```python
from build123d import *

# Parameters (mm, degrees)
SKETCH3_W                       = 0.5
SKETCH3_H                       = 1.75
SKETCH3_W_2                     = 1.75
SKETCH3_H_2                     = 0.5
BOSS_EXTRUDE1_DEPTH             = 13
BOSS_EXTRUDE1_DIRECTION_2_REACH = 27.695
SKETCH4_R                       = 0.75
CUT_EXTRUDE2_DEPTH              = 4
BOSS_EXTRUDE2_DEPTH             = 1


with BuildPart() as part:
    # Sketch1 → Revolve1 (revolve)
    with BuildSketch(Plane(origin=(0, 0, 0), x_dir=(0, 0, -1), z_dir=(1, 0, 0))):
        with BuildLine():
            ThreePointArc((-3.5, 4), (-2.474873734, 1.525126266), (0, 0.5))
            Line((0, 0.5), (0, 0))
            Line((0, 0), (0, -8.5))
            Line((0, -8.5), (0, -14.5))
            ThreePointArc((0, -14.5), (-2.956795679, -12.007305936), (-1, -8.671572875))
            Line((-1, -8.671572875), (-1, 0.127016654))
            ThreePointArc((-1, 0.127016654), (-2.197145125, 0.657463044), (-3.158848322, 1.546089391))
            Line((-3.158848322, 1.546089391), (-15, 3))
            Line((-15, 3), (-15, 4))
            Line((-15, 4), (-4, 4))
            Line((-4, 4), (-3.5, 4))
        make_face()
    revolve(axis=Axis((0, 10.634252877, 0), (0, 1, 0)))

    # Sketch3 → Boss-Extrude1 (add)
    with BuildSketch(Plane(origin=(0, 0, 0), x_dir=(1, 0, 0), z_dir=(0, 1, 0))):
        with Locations((0, 1.125)):
            Rectangle(SKETCH3_W, SKETCH3_H)
        with Locations((-1.125, 0)):
            Rectangle(SKETCH3_W_2, SKETCH3_H_2)
        with Locations((1.125, 0)):
            Rectangle(SKETCH3_W_2, SKETCH3_H_2)
        with Locations((0, -1.125)):
            Rectangle(SKETCH3_W, SKETCH3_H)
    extrude(amount=-BOSS_EXTRUDE1_DEPTH)

    # Sketch3 → Boss-Extrude1 direction 2 (add, up to next)
    with BuildSketch(Plane(origin=(0, 0, 0), x_dir=(1, 0, 0), z_dir=(0, 1, 0)), mode=Mode.PRIVATE) as boss_extrude1_direction_2_sk1:
        with Locations((0, 1.125)):
            Rectangle(SKETCH3_W, SKETCH3_H)
    boss_extrude1_direction_2_tool1 = extrude(boss_extrude1_direction_2_sk1.sketch, amount=BOSS_EXTRUDE1_DIRECTION_2_REACH, mode=Mode.PRIVATE) - part.part
    # Sketch3 → Boss-Extrude1 direction 2 (add, up to next)
    with BuildSketch(Plane(origin=(0, 0, 0), x_dir=(1, 0, 0), z_dir=(0, 1, 0)), mode=Mode.PRIVATE) as boss_extrude1_direction_2_sk2:
        with Locations((-1.125, 0)):
            Rectangle(SKETCH3_W_2, SKETCH3_H_2)
    boss_extrude1_direction_2_tool2 = extrude(boss_extrude1_direction_2_sk2.sketch, amount=BOSS_EXTRUDE1_DIRECTION_2_REACH, mode=Mode.PRIVATE) - part.part
    # Sketch3 → Boss-Extrude1 direction 2 (add, up to next)
    with BuildSketch(Plane(origin=(0, 0, 0), x_dir=(1, 0, 0), z_dir=(0, 1, 0)), mode=Mode.PRIVATE) as boss_extrude1_direction_2_sk3:
        with Locations((1.125, 0)):
            Rectangle(SKETCH3_W_2, SKETCH3_H_2)
    boss_extrude1_direction_2_tool3 = extrude(boss_extrude1_direction_2_sk3.sketch, amount=BOSS_EXTRUDE1_DIRECTION_2_REACH, mode=Mode.PRIVATE) - part.part
    # Sketch3 → Boss-Extrude1 direction 2 (add, up to next)
    with BuildSketch(Plane(origin=(0, 0, 0), x_dir=(1, 0, 0), z_dir=(0, 1, 0)), mode=Mode.PRIVATE) as boss_extrude1_direction_2_sk4:
        with Locations((0, -1.125)):
            Rectangle(SKETCH3_W, SKETCH3_H)
    boss_extrude1_direction_2_tool4 = extrude(boss_extrude1_direction_2_sk4.sketch, amount=BOSS_EXTRUDE1_DIRECTION_2_REACH, mode=Mode.PRIVATE) - part.part
    add(boss_extrude1_direction_2_tool1.solids().sort_by_distance((0, 0, -1.125))[0])
    add(boss_extrude1_direction_2_tool2.solids().sort_by_distance((-1.125, 0, 0))[0])
    add(boss_extrude1_direction_2_tool3.solids().sort_by_distance((1.125, 0, 0))[0])
    add(boss_extrude1_direction_2_tool4.solids().sort_by_distance((0, 0, 1.125))[0])

    # Sketch4 → Cut-Extrude2 (cut)
    with BuildSketch(Plane(origin=(0, 4, 0), x_dir=(1, 0, 0), z_dir=(0, 1, 0))):
        with BuildLine():
            Line((-1.190417877, 5.369628039), (-2.813714981, 12.691848093))
            ThreePointArc((-2.813714981, 12.691848093), (-9.192388155, 9.192388155), (-12.691848093, 2.813714981))
            Line((-12.691848093, 2.813714981), (-5.369628039, 1.190417877))
            ThreePointArc((-5.369628039, 1.190417877), (-3.889087297, 3.889087297), (-1.190417877, 5.369628039))
        make_face()
        with BuildLine():
            Line((-5.369628039, -1.190417877), (-12.691848093, -2.813714981))
            ThreePointArc((-12.691848093, -2.813714981), (-9.192388155, -9.192388155), (-2.813714981, -12.691848093))
            Line((-2.813714981, -12.691848093), (-1.190417877, -5.369628039))
            ThreePointArc((-1.190417877, -5.369628039), (-3.889087297, -3.889087297), (-5.369628039, -1.190417877))
        make_face()
        with BuildLine():
            ThreePointArc((2.813714981, -12.691848093), (9.192388155, -9.192388155), (12.691848093, -2.813714981))
            Line((12.691848093, -2.813714981), (5.369628039, -1.190417877))
            ThreePointArc((5.369628039, -1.190417877), (3.889087297, -3.889087297), (1.190417877, -5.369628039))
            Line((1.190417877, -5.369628039), (2.813714981, -12.691848093))
        make_face()
        with BuildLine():
            ThreePointArc((12.691848093, 2.813714981), (9.192388155, 9.192388155), (2.813714981, 12.691848093))
            Line((2.813714981, 12.691848093), (1.190417877, 5.369628039))
            ThreePointArc((1.190417877, 5.369628039), (3.889087297, 3.889087297), (5.369628039, 1.190417877))
            Line((5.369628039, 1.190417877), (12.691848093, 2.813714981))
        make_face()
        with Locations(Location((-13, 0, 0), (0, 0, 134.983865121))):
            Circle(SKETCH4_R)
        with Locations(Location((-10, 0, 0), (0, 0, 135.012139771))):
            Circle(SKETCH4_R)
        with Locations(Location((0, 10, 0), (0, 0, 270))):
            Circle(SKETCH4_R)
        with Locations(Location((0, 13, 0), (0, 0, 270))):
            Circle(SKETCH4_R)
        with Locations(Location((0, -10, 0), (0, 0, 135.918159621))):
            Circle(SKETCH4_R)
        with Locations(Location((0, -13, 0), (0, 0, 135.875962229))):
            Circle(SKETCH4_R)
        with Locations(Location((10, 0, 0), (0, 0, 270))):
            Circle(SKETCH4_R)
        with Locations(Location((13, 0, 0), (0, 0, 270))):
            Circle(SKETCH4_R)
    extrude(amount=-CUT_EXTRUDE2_DEPTH, mode=Mode.SUBTRACT)

    # Sketch5 → Boss-Extrude2 (add)
    with BuildSketch(Plane(origin=(0, 4, 0), x_dir=(1, 0, 0), z_dir=(0, 1, 0))):
        with BuildLine():
            ThreePointArc((-11.290112025, 9.875898463), (-10.606601718, 10.606601718), (-9.875898463, 11.290112025))
            Line((-9.875898463, 11.290112025), (-15, 15))
            Line((-15, 15), (-11.290112025, 9.875898463))
        make_face()
        with BuildLine():
            Line((15, 15), (9.875898463, 11.290112025))
            ThreePointArc((9.875898463, 11.290112025), (10.606601718, 10.606601718), (11.290112025, 9.875898463))
            Line((11.290112025, 9.875898463), (15, 15))
        make_face()
        with BuildLine():
            ThreePointArc((11.290112025, -9.875898463), (10.606601718, -10.606601718), (9.875898463, -11.290112025))
            Line((9.875898463, -11.290112025), (15, -15))
            Line((15, -15), (11.290112025, -9.875898463))
        make_face()
        with BuildLine():
            ThreePointArc((-9.875898463, -11.290112025), (-10.606601718, -10.606601718), (-11.290112025, -9.875898463))
            Line((-11.290112025, -9.875898463), (-15, -15))
            Line((-15, -15), (-9.875898463, -11.290112025))
        make_face()
    extrude(amount=-BOSS_EXTRUDE2_DEPTH)


solid = part.part
```
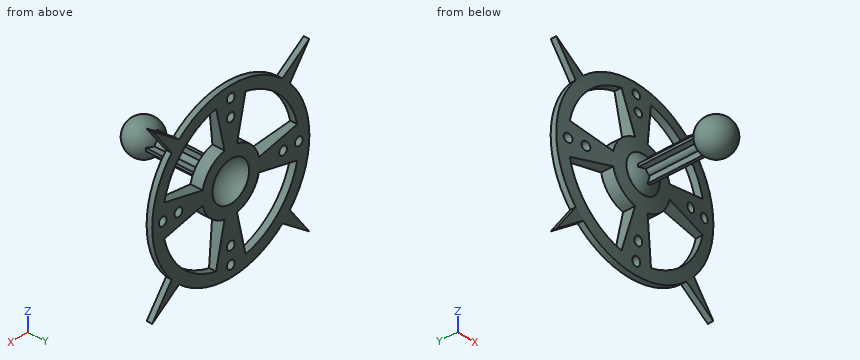
Verification items for the finished model (mm, model axes). Coordinates: 2 decimals unless noted, no trailing zeros. Loops run counter-clockwise (first coordinate to the right, second up) from the corner with the lowest first, then second, coordinate; pieces in that order, holes last. Notation, with made-up numbers: (15.5, 6) -> (37.5, 6) arc R5 ccw to (37.5, 12) -> close; hole circle Ø8 at (78.5, 79). An arc over 180 degrees is marked (long way). Answer in a Markdown table with one row per item. Add a question column.
1. Material ranges on probe 1 along Z at (x, y) = (-13, 3.3); probe 2 along X at (y, z) = (3.1, 10); probe 3 along X at (y, z) = (2.75, 0), recorded low to high. Write a range as [from, to].
2. Section check B-B, the plane z = 6.5. Give the number of separate pieces and of enclosed holes in the cut face, then the cut area to 3 significant figures.
3. Section check A-A, the plane y = -7. Enter the section's corners in (x, z), then the cut area to 3 significant figures.
4. Depth check by flat-ended pin: P1, Ø0.5, axis at x = 1.5, y = -4.5, coming from the +Z side; P2, Ø5.5, axis at x = -12, z = 13.5, coming from the -Y side; P3, Ø0.8, axis at y = -2.5, z = 1.5, coming from the +X side. Enter the tip coordinate at first touch or a pass-through.
Derived:
| question | item | result |
|---|---|---|
| 1 | probe 1 | z = [-13.55, -12.24], [-7.48, -0.75], [0.75, 7.48], [12.24, 13.55] |
| 1 | probe 2 | x = [-11.38, -8.31], [-2.22, -0.75], [0.75, 2.22], [8.31, 11.38] |
| 1 | probe 3 | x = [-12.25, -10.75], [-9.25, -3.27], [3.27, 9.25], [10.75, 12.25] |
| 2 | separate pieces | 3 |
| 2 | enclosed holes | 0 |
| 2 | area | 11.0 mm² |
| 3 | outline | (-2, -0.25) -> (-0.97, -0.25) arc R1 ccw to (-0.25, -0.97) -> (-0.25, -2) -> (0.25, -2) -> (0.25, -0.97) arc R1 ccw to (0.97, -0.25) -> (2, -0.25) -> (2, 0.25) -> (0.97, 0.25) arc R1 ccw to (0.25, 0.97) -> (0.25, 2) -> (-0.25, 2) -> (-0.25, 0.97) arc R1 ccw to (-0.97, 0.25) -> (-2, 0.25) -> close |
| 3 | area | 5.16 mm² |
| 4 | P1 | stops at z = 0.25 |
| 4 | P2 | stops at y = 3 |
| 4 | P3 | stops at x = 0.25 |
